Read the model definition and answer for the solid it produces. Units are mm, in the model's axes. Face numbers are marked on the shaded views. Coordinates: 2 decimals unless noted, no trailing zeros. Order: outer loops, then holes, each group sorted by start corner. A loop starts at its lowest first (then second) coordinate and runs counter-clockwise, first axis right, second up. Notation, with made-up numbers: (-23.75, -27) -> (14.25, -27) arc R12 cw to (14.25, -8) -> close; hole circle Ø5 at (72.25, -33.5). An arc over 180 degrees is marked (long way). Return JSON: item names as keys, results as strings. Group by question number.
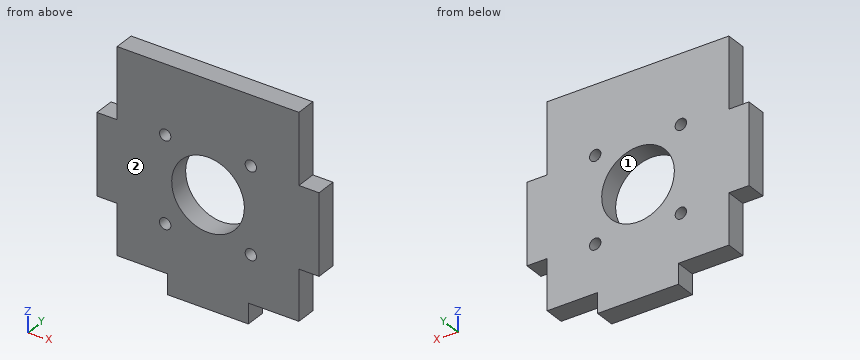
```python
from build123d import *

# Parameters (mm, degrees)
SKETCH1_R      = 11.43
SKETCH1_R_2    = 1.7859375
EXTRUDE1_DEPTH = 6.35


with BuildPart() as part:
    # Sketch1 → Extrude1 (new body)
    with BuildSketch(Plane(origin=(0, 0, 0), x_dir=(1, 0, 0), z_dir=(0, 1, 0))):
        Polygon((6.35, 47.625), (0, 47.625), (0, 22.225), (6.35, 22.225), (6.35, 0), (63.5, 0), (63.5, 22.225), (69.85, 22.225), (69.85, 47.625), (63.5, 47.625), (63.5, 63.5), (47.625, 63.5), (47.625, 69.85), (22.225, 69.85), (22.225, 63.5), (6.35, 63.5), align=None)
        with Locations(Location((34.925, 35.052, 0), (0, 0, 270))):
            Circle(SKETCH1_R, mode=Mode.SUBTRACT)
        with Locations(Location((21.454615818, 48.522384182, 0), (0, 0, 270))):
            Circle(SKETCH1_R_2, mode=Mode.SUBTRACT)
        with Locations(Location((48.395384182, 48.522384182, 0), (0, 0, 270))):
            Circle(SKETCH1_R_2, mode=Mode.SUBTRACT)
        with Locations(Location((48.395384182, 21.581615818, 0), (0, 0, 270))):
            Circle(SKETCH1_R_2, mode=Mode.SUBTRACT)
        with Locations(Location((21.454615818, 21.581615818, 0), (0, 0, 270))):
            Circle(SKETCH1_R_2, mode=Mode.SUBTRACT)
    extrude(amount=EXTRUDE1_DEPTH)


solid = part.part
```
1. Straight lines are drawn through the part: L1, parallel to Z at x = 47.5, y = 4.5; L2, parallel to X at y = 2, z = -59; L3, parallel to X at y = 6.25, z = -32.5. For each, find the intervals that lie inside material, in ascending order.
2. Find section B-B on y = 1.5. Determine the outline of the cut face in (x, z) (3 decimals).
3. Find section A-A on z = -21. Determine the outline of the cut face in (x, y), and give its area (3 significant figures).
4. Find section C-C on z = -38. Determine the outline of the cut face in (x, y), and give its area (3 significant figures).
5. Given pin 1 (3 mm diameter, centred on x = 2, y = 4, fed in from -Z) (3 decimals); pin 2 (1.5 mm diameter, centred on y = 5, z = -19.5, fed in from -X); pin 3 (1.9 mm diameter, centred on y = 3, z = -9, fed in from +X), each flat-ended and moving along its own axis, determine where each tip first touches the part or whether it passes through.
6. For a pull along X with two mould halves and no side action, classify the marked faces 1 and 2 as released by +X, released by -X, zero draft, split by the parting line, or undercut.
7. Find section D-D on x = 59.5. Determine the outline of the cut face in (y, z).
Result:
{
 "1": {"L1": "-69.85 to -50.07, -46.98 to -23.13, -20.04 to 0", "L2": "6.35 to 63.5", "L3": "0 to 23.78, 46.07 to 69.85"},
 "2": {"outline": "(0, -47.625) -> (6.35, -47.625) -> (6.35, -63.5) -> (22.225, -63.5) -> (22.225, -69.85) -> (47.625, -69.85) -> (47.625, -63.5) -> (63.5, -63.5) -> (63.5, -47.625) -> (69.85, -47.625) -> (69.85, -22.225) -> (63.5, -22.225) -> (63.5, 0) -> (6.35, 0) -> (6.35, -22.225) -> (0, -22.225) -> close; hole circle Ø3.572 at (21.455, -48.522); hole circle Ø3.572 at (21.455, -21.582); hole circle Ø22.86 at (34.925, -35.052); hole circle Ø3.572 at (48.395, -48.522); hole circle Ø3.572 at (48.395, -21.582)"},
 "3": {"outline": "(6.35, 0) -> (19.77, 0) -> (19.77, 6.35) -> (6.35, 6.35) -> close; (23.14, 0) -> (46.71, 0) -> (46.71, 6.35) -> (23.14, 6.35) -> close; (50.08, 0) -> (63.5, 0) -> (63.5, 6.35) -> (50.08, 6.35) -> close", "area": "320 mm^2"},
 "4": {"outline": "(0, 0) -> (23.88, 0) -> (23.88, 6.35) -> (0, 6.35) -> close; (45.97, 0) -> (69.85, 0) -> (69.85, 6.35) -> (45.97, 6.35) -> close", "area": "303 mm^2"},
 "5": {"pin 1": "z = -47.625", "pin 2": "x = 6.35", "pin 3": "x = 63.5"},
 "6": {"face 1": "undercut", "face 2": "zero draft"},
 "7": {"outline": "(0, -63.5) -> (6.35, -63.5) -> (6.35, 0) -> (0, 0) -> close"}
}
